Here's how the part is built. I have some questions about the finished solid (model axes, mm). A direction names the side the tool comes from. Round coordinates to 2 decimals unless told otherwise and drop trailing zeros. Loops run counter-clockwise (first coordinate to the right, second up) from the corner with the lowest first, then second, coordinate; pieces in that order, holes last. Notation, with made-up numbers: (10.5, -34) - (66.5, -34) arc R35 ccw to (66.5, 0) - close; hole circle Ø8 at (-34.75, 88). An arc over 180 degrees is marked (long way). Answer as a JSON object with one key per item and string values. Group by question number.
1) I want a section at B-B, the plane y = 10.5. Please give me the cut outline in (x, z).
2) Which directions (+Z, -Z, +X, -X, +Y, -Y) give clear straight access to the entire face, cutting with the end or side of a thin tool? Please do faces 5 (the face through (-42.594, 1.479, -55.55)), 6 (the face through (1.627, 8.577, 122.394)).
3) If I drill on line 1 along X through (y, z) = (6.75, 0); line 2 along Y through (x, z) = (79, -82); line 3 along X through (y, z) = (6.75, 9), over which ranges is the centre line in solid material (lowest first)? Write a range as [from, to].
4) I want a section at C-C, the plane x = 0. Please give me the cut outline in (y, z).
5) Will these pins go through, and if not, where does the flat tip stop? P1, Ø20, axis at x = -110, z = 0, coming from the -Y side (3 decimals); P2, Ø8, axis at x = -58, y = 2, coming from the +Z side; P3, Ø1, axis at x = 21, y = 6, coming from the -Z side; P4, Ø1.5, axis at y = 4, z = -47.5, coming from the +X side.
6) If we mould it in two halves opening along Z, with no side actions, what happens to faces 1 (the face through (-53.692, 7.098, -11.923)), 2 (the face through (2, 14, -58)), 3 (the face through (-1.627, 8.577, -122.394)), 4 (the face through (-82.15, 8.42, -107.13))? For each: pulls with the +Z half, pulls with the -Z half, needs draft (parallel to the pull), parting line crosses it, or undercut.
7) I want a section at A-A, the plane z = 0. Please give me the cut outline in (x, y).
8) I want a section at D-D, the plane z = -41.5. Please give me the cut outline in (x, y).
from build123d import *

# Parameters (mm, degrees)
F3_D            = 25
F3_COPIES_COUNT = 4


# Not quite as in the source:
# - a pattern or mirror of a feature is missing from the dataset's text; its kind, count and spacing are read off the source's solid


with BuildPart() as f1:
    # F0 (on Right) → F1 (revolve)
    with BuildSketch(Plane.YZ):
        Polygon((0, 70), (0, 55), (14, 55), (14, 135), (3, 135), (3, 70), align=None)
    revolve(axis=Axis((0, 31.8317301571, 0), (0, 1, 0)))

    # F3 (through all)
    with Locations(Plane.XZ.offset(-3)):
        with Locations((0, 110)):
            f3 = Hole(F3_D / 2)

    # F3_copies: F3 ×4 about axis
    f3_copies_axis = Axis((0, 0, 0), (0, 1, 0))
    for i in range(1, F3_COPIES_COUNT):
        add(f3.rotate(f3_copies_axis, i * 360 / F3_COPIES_COUNT), mode=Mode.SUBTRACT)


solid = f1.part
Outcome:
{
 "1": {"outline": "circle Ø270 at (0, 0); hole circle Ø25 at (-110, 0); hole circle Ø110 at (0, 0); hole circle Ø25 at (0, -110); hole circle Ø25 at (0, 110); hole circle Ø25 at (110, 0)"},
 "2": {"face 5": "-Y", "face 6": "+Y, -Y"},
 "3": {"line 1": "[-135, -122.5], [-97.5, -55], [55, 97.5], [122.5, 135]", "line 2": "[3, 14]", "line 3": "[-134.7, -118.67], [-101.33, -54.26], [54.26, 101.33], [118.67, 134.7]"},
 "4": {"outline": "(0, -70) - (3, -70) - (3, -97.5) - (14, -97.5) - (14, -55) - (0, -55) - close; (0, 55) - (14, 55) - (14, 97.5) - (3, 97.5) - (3, 70) - (0, 70) - close; (3, -135) - (14, -135) - (14, -122.5) - (3, -122.5) - close; (3, 122.5) - (14, 122.5) - (14, 135) - (3, 135) - close"},
 "5": {"P1": "through", "P2": "z = 123.67", "P3": "z = -133.43", "P4": "x = 126.65"},
 "6": {"face 1": "undercut", "face 2": "needs draft", "face 3": "undercut", "face 4": "parting line crosses it"},
 "7": {"outline": "(-135, 3) - (-122.5, 3) - (-122.5, 14) - (-135, 14) - close; (-97.5, 3) - (-70, 3) - (-70, 0) - (-55, 0) - (-55, 14) - (-97.5, 14) - close; (55, 0) - (70, 0) - (70, 3) - (97.5, 3) - (97.5, 14) - (55, 14) - close; (122.5, 3) - (135, 3) - (135, 14) - (122.5, 14) - close"},
 "8": {"outline": "(-128.46, 3) - (-56.37, 3) - (-56.37, 0) - (-36.09, 0) - (-36.09, 14) - (-128.46, 14) - close; (36.09, 0) - (56.37, 0) - (56.37, 3) - (128.46, 3) - (128.46, 14) - (36.09, 14) - close"}
}
